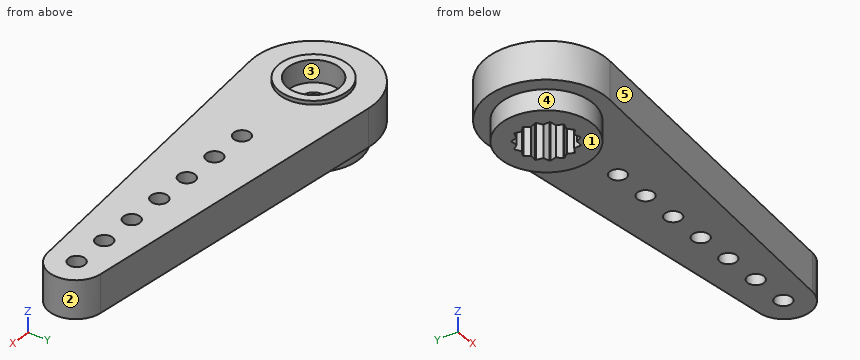
```python
from build123d import *

# Parameters (mm, degrees)
BOSS_EXTRUDE1_DEPTH = 5
CUT_EXTRUDE1_REACH  = 49.569
SKETCH2_R           = 1.5
SKETCH3_R           = 3.4
CUT_EXTRUDE2_DEPTH  = 2.4
BOSS_EXTRUDE2_START = 0.5
SKETCH4_R           = 4.5
SKETCH4_R_2         = 3.4
BOSS_EXTRUDE2_DEPTH = 0.5
SKETCH6_R           = 6
SKETCH6_R_2         = 1.5
BOSS_EXTRUDE3_DEPTH = 2.7
SKETCH7_R           = 3.75
CUT_EXTRUDE4_DEPTH  = 5
BOSS_EXTRUDE4_DEPTH = 5
CIRPATTERN2_COUNT   = 15
CUT_EXTRUDE5_REACH  = 49.928
SKETCH10_R          = 1.09


with BuildPart() as part:
    # Sketch1 → Boss-Extrude1 (new body)
    with BuildSketch(Plane.XY):
        with BuildLine():
            Line((0.788456111, 7.810303257), (43.485538544, 3.5))
            ThreePointArc((43.485538544, 3.5), (46.65, 0), (43.485538544, -3.5))
            Line((43.485538544, -3.5), (0.788456111, -7.810303257))
            ThreePointArc((0.788456111, -7.810303257), (-7.85, 0), (0.788456111, 7.810303257))
        make_face()
    extrude(amount=BOSS_EXTRUDE1_DEPTH)

    # Sketch2 → Cut-Extrude1 (cut, up to next)
    with BuildSketch(Plane.XY.offset(5), mode=Mode.PRIVATE) as cut_extrude1_sk1:
        Circle(SKETCH2_R)
    cut_extrude1_tool1 = extrude(cut_extrude1_sk1.sketch, amount=-CUT_EXTRUDE1_REACH, mode=Mode.PRIVATE) & part.part
    add(cut_extrude1_tool1.solids().sort_by_distance((0, 0, 5))[0], mode=Mode.SUBTRACT)

    # Sketch3 → Cut-Extrude2 (cut)
    with BuildSketch(Plane.XY.offset(5)):
        Circle(SKETCH3_R)
    extrude(amount=-CUT_EXTRUDE2_DEPTH, mode=Mode.SUBTRACT)

    # Sketch4 → Boss-Extrude2 (add)
    with BuildSketch(Plane.XY.offset(5).offset(BOSS_EXTRUDE2_START)):
        Circle(SKETCH4_R)
        Circle(SKETCH4_R_2, mode=Mode.SUBTRACT)
    extrude(amount=-BOSS_EXTRUDE2_DEPTH)

    # Sketch6 → Boss-Extrude3 (add)
    with BuildSketch(Plane(origin=(0, 0, 0), x_dir=(-1, 0, 0), z_dir=(0, 0, -1))):
        with Locations(Location((0, 0, 0), (0, 0, 180))):
            Circle(SKETCH6_R)
        with Locations(Location((0, 0, 0), (0, 0, 180))):
            Circle(SKETCH6_R_2, mode=Mode.SUBTRACT)
    extrude(amount=BOSS_EXTRUDE3_DEPTH)

    # Sketch7 → Cut-Extrude4 (cut)
    with BuildSketch(Plane(origin=(0, 0, -2.7), x_dir=(-1, 0, 0), z_dir=(0, 0, -1))):
        Circle(SKETCH7_R)
    extrude(amount=-CUT_EXTRUDE4_DEPTH, mode=Mode.SUBTRACT)

    # Sketch8 → Boss-Extrude4 (add)
    with BuildSketch(Plane(origin=(0, 0, -2.7), x_dir=(-1, 0, 0), z_dir=(0, 0, -1))):
        with BuildLine():
            Line((-0.738744308, 3.676514225), (0, 3.25))
            Line((0, 3.25), (0.738744308, 3.676514225))
            ThreePointArc((0.738744308, 3.676514225), (0, 3.75), (-0.738744308, 3.676514225))
        make_face()
    boss_extrude4 = extrude(amount=-BOSS_EXTRUDE4_DEPTH)

    # CirPattern2: Boss-Extrude4 ×15 about axis
    cirpattern2_axis = Axis((0, 0, 0), (0, 0, 1))
    for i in range(1, CIRPATTERN2_COUNT):
        add(boss_extrude4.rotate(cirpattern2_axis, i * 360 / CIRPATTERN2_COUNT))

    # Sketch10 → Cut-Extrude5 (cut, up to next)
    with BuildSketch(Plane.XY.offset(5), mode=Mode.PRIVATE) as cut_extrude5_sk1:
        with Locations((43, 0)):
            Circle(SKETCH10_R)
    cut_extrude5_tool1 = extrude(cut_extrude5_sk1.sketch, amount=-CUT_EXTRUDE5_REACH, mode=Mode.PRIVATE) & part.part
    # Sketch10 → Cut-Extrude5 (cut, up to next)
    with BuildSketch(Plane.XY.offset(5), mode=Mode.PRIVATE) as cut_extrude5_sk2:
        with Locations((38, 0)):
            Circle(SKETCH10_R)
    cut_extrude5_tool2 = extrude(cut_extrude5_sk2.sketch, amount=-CUT_EXTRUDE5_REACH, mode=Mode.PRIVATE) & part.part
    # Sketch10 → Cut-Extrude5 (cut, up to next)
    with BuildSketch(Plane.XY.offset(5), mode=Mode.PRIVATE) as cut_extrude5_sk3:
        with Locations((33, 0)):
            Circle(SKETCH10_R)
    cut_extrude5_tool3 = extrude(cut_extrude5_sk3.sketch, amount=-CUT_EXTRUDE5_REACH, mode=Mode.PRIVATE) & part.part
    # Sketch10 → Cut-Extrude5 (cut, up to next)
    with BuildSketch(Plane.XY.offset(5), mode=Mode.PRIVATE) as cut_extrude5_sk4:
        with Locations((28, 0)):
            Circle(SKETCH10_R)
    cut_extrude5_tool4 = extrude(cut_extrude5_sk4.sketch, amount=-CUT_EXTRUDE5_REACH, mode=Mode.PRIVATE) & part.part
    # Sketch10 → Cut-Extrude5 (cut, up to next)
    with BuildSketch(Plane.XY.offset(5), mode=Mode.PRIVATE) as cut_extrude5_sk5:
        with Locations((23, 0)):
            Circle(SKETCH10_R)
    cut_extrude5_tool5 = extrude(cut_extrude5_sk5.sketch, amount=-CUT_EXTRUDE5_REACH, mode=Mode.PRIVATE) & part.part
    # Sketch10 → Cut-Extrude5 (cut, up to next)
    with BuildSketch(Plane.XY.offset(5), mode=Mode.PRIVATE) as cut_extrude5_sk6:
        with Locations((18, 0)):
            Circle(SKETCH10_R)
    cut_extrude5_tool6 = extrude(cut_extrude5_sk6.sketch, amount=-CUT_EXTRUDE5_REACH, mode=Mode.PRIVATE) & part.part
    # Sketch10 → Cut-Extrude5 (cut, up to next)
    with BuildSketch(Plane.XY.offset(5), mode=Mode.PRIVATE) as cut_extrude5_sk7:
        with Locations((13, 0)):
            Circle(SKETCH10_R)
    cut_extrude5_tool7 = extrude(cut_extrude5_sk7.sketch, amount=-CUT_EXTRUDE5_REACH, mode=Mode.PRIVATE) & part.part
    add(cut_extrude5_tool1.solids().sort_by_distance((43, 0, 5))[0], mode=Mode.SUBTRACT)
    add(cut_extrude5_tool2.solids().sort_by_distance((38, 0, 5))[0], mode=Mode.SUBTRACT)
    add(cut_extrude5_tool3.solids().sort_by_distance((33, 0, 5))[0], mode=Mode.SUBTRACT)
    add(cut_extrude5_tool4.solids().sort_by_distance((28, 0, 5))[0], mode=Mode.SUBTRACT)
    add(cut_extrude5_tool5.solids().sort_by_distance((23, 0, 5))[0], mode=Mode.SUBTRACT)
    add(cut_extrude5_tool6.solids().sort_by_distance((18, 0, 5))[0], mode=Mode.SUBTRACT)
    add(cut_extrude5_tool7.solids().sort_by_distance((13, 0, 5))[0], mode=Mode.SUBTRACT)


solid = part.part
```
Geometry check sheet. Reference: the model listing, model coordinates, mm. Face numbers are marked on the shaded views. A direction names the side the tool comes from. Coordinates: 2 decimals unless noted, no trailing zeros. Order: outer loops, then holes, each group sorted by start corner. A loop starts at its lowest first (then second) coordinate and runs counter-clockwise, first axis right, second up. Notation, with made-up numbers: M 40.5,70.5 L 88.5,70.5 A18 cw 88.5,77.5 Z; hole C 28.25,84 d7. An arc over 180 degrees is marked long. Answer as a JSON object with one key per item and string values.
Q1. Cross-section at C-C on x = 23. Record the cut outline in (y, z).
Results are:
{"outline": "M -5.57,0 L -1.09,0 L -1.09,5 L -5.57,5 Z; M 1.09,0 L 5.57,0 L 5.57,5 L 1.09,5 Z"}
Q2. Cross-section at D-D on x = 7. Record the cut outline in (y, z), and give its area (3 significant figures).
Results are:
{"outline": "M -7.18,0 L 7.18,0 L 7.18,5 L -7.18,5 Z", "area": "71.8 mm²"}
Q3. Cross-section at A-A on x = 17.5. Record the cut outline in (y, z), and give its area (3 significant figures).
Results are:
{"outline": "M -6.12,0 L -0.97,0 L -0.97,5 L -6.12,5 Z; M 0.97,0 L 6.12,0 L 6.12,5 L 0.97,5 Z", "area": "51.5 mm²"}
Q4. Depth check by flat-ended pin: pin 1 Ø3 at (x, y) = (43, 0) entering from -Z; pin 2 Ø1 at (x, z) = (19.5, -1.5) entering from +Y; pin 3 Ø4 at (x, y) = (0, 0) entering from +Z; pin 4 Ø8 at (x, y) = (21.5, -1) entering from +Z. Enter the tip coordinate at first touch or a pass-through.
Results are:
{"pin 1": "stops at z = 0", "pin 2": "passes through", "pin 3": "stops at z = 2.6", "pin 4": "stops at z = 5"}
Q5. Scan lines: line 1 (Y direction, x = 43, z = 3); line 2 (Z direction, x = 31, y = 2); line 3 (Y direction, x = 18, z = 4). Record each from-to range of solid material in increasing order.
Results are:
{"line 1": "y = -3.55 to -1.09, 1.09 to 3.55", "line 2": "z = 0 to 5", "line 3": "y = -6.07 to -1.09, 1.09 to 6.07"}
Q6. Release check for a two-part mould opening along Y. For the marked faces 1, 2 and 3 record: released by +Y, released by -Y, zero draft, split by the parting line, or undercut.
Results are:
{"face 1": "zero draft", "face 2": "split by the parting line", "face 3": "undercut"}
Q7. Tool access check on the marked faces 4 and 5. Record the directions out of +Z, -Z, +X, -X, +Y, -Y that give a thin tool (end or side, any length) a straight path to the whole face; none if there is none.
Results are:
{"face 4": "-Z", "face 5": "+Z, -Z, +X, -Y"}
Q8. Cross-section at B-B on z = 1.75. Give the number of separate pieces and of enclosed holes in the cut face, and give its area (3 significant figures).
Results are:
{"separate pieces": "1", "enclosed holes": "8", "area": "545 mm²"}
